Build history of the part. All positions in model axes, mm. A direction names the side the tool comes from. Round coordinates to 2 decimals unless told otherwise and drop trailing zeros. One line per item, written item: value. Start each with the question number.
Item 1: Probe L1, parallel to Z at x = -14, y = -35.5; L2, parallel to Z at x = 15, y = 14.5; L3, parallel to X at y = 33, z = -66.5 (3 decimals). List the from-to ranges inside material, lowest first.
Item 2: Pin check, flat tips, straight feed: pin 1 (3 mm diameter, centred on x = 29.5, z = -37.5, fed in from -Y); pin 2 (1 mm diameter, centred on y = -28.5, z = -18, fed in from -X) (3 decimals); pin 3 (1.5 mm diameter, centred on x = 31, y = -10, fed in from -Z). Stop position of each tip, or through.
Item 3: Tool access for faces 4 (the flat face through (2.8, -35.4, 0)), 5 (the flat face through (33.15, -28.87, -37.58)), 6 (the flat face through (28.91, 33, -38.42)): list every direction of +Z, -Z, +X, -X, +Y, -Y with a clear straight run to the whole face (end or side of a thin tool).
Item 4: Band-saw the part on A-A, the plane z = -19. Give the number of separate pieces and of enclosed holes in the cut face, then the cut area to 3 significant figures.
Item 5: Two-plate mould, pull along X, no slides. Class faces 1 (the flat face through (-31.38, 35.46, -87.83)), 2 (the flat face through (40, 0, 2)), 3 (the flat face through (36, 36, -100)): +X half, -X half, draft (parallel to the pull), parting line (faces both ways), or undercut.
```python
from build123d import *

# Parameters (mm, degrees)
F0_W      = 70
F0_H      = 70
F2_W      = 80
F2_H      = 80
F5_DEPTH  = 62.8
F7_DEPTH  = 96
F8_W      = 61.5800124844
F8_H      = 61.5800124844
F9_W      = 54.7800124844
F9_H      = 54.7800124844
F11_W     = 80
F11_H     = 80
F12_DEPTH = 5
F13_R     = 5


with BuildPart() as f3:
    # F0 (on Top) → F3 section 0
    with BuildSketch(Plane.XY):
        Rectangle(F0_W, F0_H)
    # F2 (on offset) → F3 section 1
    with BuildSketch(Plane.XY.offset(-100)):
        Rectangle(F2_W, F2_H)
    loft()

    # F4 (on Front) → F5 (cut, symmetric)
    with BuildSketch(Plane.XZ):
        Polygon((-31.9900062422, -100), (31.9900062422, -100), (30.7900062422, -76), (-30.7900062422, -76), align=None)
        Polygon((27.3900062422, -8), (-27.3900062422, -8), (-30.3900062422, -68), (30.3900062422, -68), align=None)
    extrude(amount=F5_DEPTH, both=True, mode=Mode.SUBTRACT)

    # F6 (on Right) → F7 (cut, symmetric)
    with BuildSketch(Plane.YZ):
        Polygon((-31.9900062422, -100), (31.9900062422, -100), (30.7900062422, -76), (-30.7900062422, -76), align=None)
        Polygon((30.3900062422, -68), (27.3900062422, -8), (-27.3900062422, -8), (-30.3900062422, -68), align=None)
    extrude(amount=F7_DEPTH, both=True, mode=Mode.SUBTRACT)

    # F8 (on face) → F10 section 0
    with BuildSketch(Plane(origin=(0, 0, -76), x_dir=(1, 0, 0), z_dir=(0, 0, -1))):
        Rectangle(F8_W, F8_H)
    # F9 (on face) → F10 section 1
    with BuildSketch(Plane.XY):
        Rectangle(F9_W, F9_H)
    loft(mode=Mode.SUBTRACT)

    # F11 (on face) → F12 (join)
    with BuildSketch(Plane.XY):
        Rectangle(F11_W, F11_H)
    extrude(amount=F12_DEPTH)

    # F13
    f13_edges = [f3.edges().sort_by_distance(p)[0] for p in [
        (-40, 40, 2.5),
        (-40, -40, 2.5),
        (40, -40, 2.5),
        (40, 40, 2.5),
    ]]
    fillet(f13_edges, radius=F13_R)


solid = f3.part
```
Output:
1. L1: z = -76 to -68, 0 to 5
1. L2: z = 0 to 5
1. L3: x = -38.325 to -30.315, 30.315 to 38.325
2. pin 1: stops at y = -36.95
2. pin 2: stops at x = -35.925
2. pin 3: stops at z = -76
3. face 4: none
3. face 5: +X, -X
3. face 6: +Y, -Y
4. separate pieces: 4
4. enclosed holes: 0
4. area: 256 mm²
5. face 1: undercut
5. face 2: +X half
5. face 3: draft
